```python
from build123d import *

# Parameters (mm, degrees)
SKETCH1_R           = 27.5
BOSS_EXTRUDE1_DEPTH = 100
CHAMFER1_SIZE       = 7
CHAMFER1_SIZE2      = 12.124355653
CHAMFER2_SIZE       = 7
SKETCH2_R           = 18
CUT_EXTRUDE1_DEPTH  = 4
FILLET1_R           = 1
CUT_EXTRUDE2_DEPTH  = 1
SKETCH6_R           = 2
BOSS_EXTRUDE2_DEPTH = 2
FILLET2_R           = 0.5
SKETCH7_R           = 1.185349533
BOSS_EXTRUDE3_DEPTH = 0.5


with BuildPart() as part:
    # Sketch1 → Boss-Extrude1 (new body)
    with BuildSketch(Plane(origin=(0, 0, 0), x_dir=(1, 0, 0), z_dir=(0, 1, 0))):
        with Locations(Location((0, 0, 0), (0, 0, 270))):
            Circle(SKETCH1_R)
    extrude(amount=BOSS_EXTRUDE1_DEPTH)

    # Chamfer1
    chamfer1_edges = [part.edges().sort_by_distance(p)[0] for p in [
        (0, 100, -27.5),
    ]]
    chamfer1_side = [part.faces().sort_by_distance(p)[0] for p in [
        (0, 100, 0),
    ]]
    chamfer(chamfer1_edges, length=CHAMFER1_SIZE, length2=CHAMFER1_SIZE2, reference=chamfer1_side[0])

    # Chamfer2
    chamfer2_edges = [part.edges().sort_by_distance(p)[0] for p in [
        (0, 0, -27.5),
    ]]
    chamfer(chamfer2_edges, length=CHAMFER2_SIZE)

    # Sketch2 → Cut-Extrude1 (cut)
    with BuildSketch(Plane(origin=(0, 100, 0), x_dir=(1, 0, 0), z_dir=(0, 1, 0))):
        with Locations(Location((0, 0, 0), (0, 0, 270))):
            Circle(SKETCH2_R)
    extrude(amount=-CUT_EXTRUDE1_DEPTH, mode=Mode.SUBTRACT)

    # Fillet1
    fillet1_edges = [part.edges().sort_by_distance(p)[0] for p in [
        (0, 100, -18),
    ]]
    fillet(fillet1_edges, radius=FILLET1_R)

    # Sketch4 → Cut-Extrude2 (cut)
    with BuildSketch(Plane(origin=(0, 96, 0), x_dir=(1, 0, 0), z_dir=(0, 1, 0))):
        with BuildLine():
            ThreePointArc((-9.270739516, -3.897699019), (0, -15), (9.270739516, -3.897699019))
            Line((9.270739516, -3.897699019), (6.887755938, 9.248526385))
            ThreePointArc((6.887755938, 9.248526385), (0, 15), (-6.887755938, 9.248526385))
            Line((-6.887755938, 9.248526385), (-9.270739516, -3.897699019))
        make_face()
    extrude(amount=-CUT_EXTRUDE2_DEPTH, mode=Mode.SUBTRACT)

    # Sketch6 → Boss-Extrude2 (add)
    # profile 1 of 2: a face of its own
    with BuildSketch(Plane(origin=(0, 95, 0), x_dir=(1, 0, 0), z_dir=(0, 1, 0))):
        with BuildLine():
            Line((-5.5, 8), (-5.5, 0))
            ThreePointArc((-5.5, 0), (0, -5.5), (5.5, 0))
            Line((5.5, 0), (5.5, 8))
            ThreePointArc((5.5, 8), (0, 13.5), (-5.5, 8))
        make_face()
        with BuildLine():
            Line((3.872983346, -1), (1.732050808, -1))
            ThreePointArc((1.732050808, -1), (0, -2), (-1.732050808, -1))
            Line((-1.732050808, -1), (-3.872983346, -1))
            ThreePointArc((-3.872983346, -1), (0, 4), (3.872983346, -1))
        make_face(mode=Mode.SUBTRACT)
        with BuildLine():
            ThreePointArc((-0.824231798, 5.146617712), (-3.677614086, 8), (-0.824231798, 10.853382288))
            Line((-0.824231798, 10.853382288), (0.824231798, 10.853382288))
            ThreePointArc((0.824231798, 10.853382288), (3.677614086, 8), (0.824231798, 5.146617712))
            Line((0.824231798, 5.146617712), (-0.824231798, 5.146617712))
        make_face(mode=Mode.SUBTRACT)
    # profile 2 of 2: a face of its own
    with BuildSketch(Plane(origin=(0, 95, 0), x_dir=(1, 0, 0), z_dir=(0, 1, 0))):
        Circle(SKETCH6_R)
    extrude(amount=BOSS_EXTRUDE2_DEPTH)

    # Fillet2
    fillet2_edges = [part.edges().sort_by_distance(p)[0] for p in [
        (-3.872983346, 96, 1),
        (3.872983346, 96, 1),
        (1.732050808, 96, 1),
        (-1.732050808, 96, 1),
    ]]
    fillet(fillet2_edges, radius=FILLET2_R)

    # Sketch7 → Boss-Extrude3 (add)
    with BuildSketch(Plane(origin=(0, 97, 0), x_dir=(1, 0, 0), z_dir=(0, 1, 0))):
        with Locations(Location((0, 0, 0), (0, 0, 270))):
            Circle(SKETCH7_R)
    extrude(amount=BOSS_EXTRUDE3_DEPTH)


solid = part.part
```
Source: CAD feature listing. Evaluate the final solid. Frame: model axes, mm. A direction names the side the tool comes from. Give positions to 0.01 mm unless a question says otherwise; leave off trailing zeros. Order: outer loops, then holes, each group sorted by start corner. A loop starts at its lowest first (then second) coordinate and runs counter-clockwise, first axis right, second up.
(1) Access query for faces 4 (the face through (-1.3, 97, -4.1)), 5 (the face through (-24.397, 46.872, 12.69)). Directions: +Z, -Z, +X, -X, +Y, -Y. A direction counts if a zero-diameter tool reaches every point of the face in a straight line with its end or side. Return the directions, or none.
(2) Contact query for flat-ended pins moving along their axis: P1, Ø4, axis at y = 10, z = 3, coming from the +X side; P2, Ø3, axis at x = -12.5, z = -9, coming from the -Y side; P3, Ø1, axis at y = 25, z = 4, coming from the -X side; P4, Ø0.7, axis at x = 0.5, z = 0.5, coming from the +Y side. Output: stop coordinate, or through.
(3) Pull-direction query (Z, two-part tool) for faces 1 (the face through (0.1, 95.5, -15)), 2 (the face through (-20.44, 99.24, -4.54)), 3 (the face through (-14, 100, 14)); classes: +Z half, -Z half, draft (parallel to the pull), parting line (faces both ways), or undercut.
(4) Material intervals for line 1 along X through (y, z) = (97.15, 0); line 2 along Z through (x, y) = (0, 95.4); line 3 along X through (y, z) = (96.45, 0), sorted ascending.
(5) Section query A-A (y = 63). Return the cut outline in (x, z), plus the area to 3 significant figures.
Outcome:
1. face 4: +Y
1. face 5: +Y, -Y
2. P1: stops at x = 27.48
2. P2: stops at y = 0
2. P3: stops at x = -27.28
2. P4: stops at y = 97.5
3. face 1: undercut
3. face 2: parting line
3. face 3: draft
4. line 1: x = -22.15 to -18, -1.19 to 1.19, 18 to 22.15
4. line 2: z = -23.16 to -15, -13.5 to -10.85, -5.15 to -4, -2 to 5.5, 15 to 23.16
4. line 3: x = -22.55 to -18, -5.5 to -4, -2 to 2, 4 to 5.5, 18 to 22.55
5. outline: circle Ø55 at (0, 0)
5. area: 2,380 mm2
